Source: CAD feature listing. Evaluate the final solid. Frame: model axes, mm. Give positions to 0.01 mm unless a question says otherwise; leave off trailing zeros. Write each loop counter-clockwise with the first axis right and the second up, starting at its lowest first coordinate (ties: lowest second). Pieces come first, ordered by that corner, then holes. Notation, with made-up numbers: (-2, 9.25) - (4, 9.25) arc R9 ccw to (4, 17.25) - close; hole circle Ø10 at (-1, -20). An arc over 180 degrees is marked (long way). One line per question, with ' | ' between items. Start each with the question number.
(1) Ray query, line 1 (Z direction, x = 254.5, y = 0.7); line 2 (Z direction, x = 114, y = 0.5); line 3 (Z direction, x = 36, y = 0.6). Return the intervals inside material, ascending. Write a range as [from, to].
(2) Section A-A, the plane x = 193. Return loops of the section in (y, z).
(3) Section B-B, the plane y = 1.6. State how many separate pieces and enclosed holes the cut face has, plus the area to 3 significant figures.
```python
from build123d import *

# Parameters (mm, degrees)
SKETCH_1_R      = 1.5
SKETCH_1_W      = 18.5
SKETCH_1_H      = 18.5
SKETCH_1_W_2    = 17
SKETCH_1_H_2    = 17
EXTRUDE_1_DEPTH = 2


with BuildPart() as part:
    # 草图1 → 凸台-拉伸1 (new body)
    with BuildSketch(Plane(origin=(0, 0, 0), x_dir=(1, 0, 0), z_dir=(0, 1, 0))):
        with BuildLine():
            Line((10, 0), (136.884360712, 0))
            ThreePointArc((136.884360712, 0), (137.900113715, -0.277140216), (138.634360712, -1.031754163))
            Line((138.634360712, -1.031754163), (139.429147615, -2.468245837))
            ThreePointArc((139.429147615, -2.468245837), (140.163394612, -3.222859784), (141.179147615, -3.5))
            Line((141.179147615, -3.5), (143.5, -3.5))
            Line((143.5, -3.5), (166.5, -3.5))
            Line((166.5, -3.5), (168.820852385, -3.5))
            ThreePointArc((168.820852385, -3.5), (169.836605388, -3.222859784), (170.570852385, -2.468245837))
            Line((170.570852385, -2.468245837), (171.365639288, -1.031754163))
            ThreePointArc((171.365639288, -1.031754163), (172.099886285, -0.277140216), (173.115639288, 0))
            Line((173.115639288, 0), (300, 0))
            ThreePointArc((300, 0), (307.071067812, -2.928932188), (310, -10))
            Line((310, -10), (310, -210))
            ThreePointArc((310, -210), (307.071067812, -217.071067812), (300, -220))
            Line((300, -220), (10, -220))
            ThreePointArc((10, -220), (2.928932188, -217.071067812), (0, -210))
            Line((0, -210), (0, -10))
            ThreePointArc((0, -10), (2.928932188, -2.928932188), (10, 0))
        make_face()
        with Locations(Location((14, -14, 0), (0, 0, 270))):
            Circle(SKETCH_1_R, mode=Mode.SUBTRACT)
        with Locations(Location((14, -206, 0), (0, 0, 270))):
            Circle(SKETCH_1_R, mode=Mode.SUBTRACT)
        with Locations(Location((296, -206, 0), (0, 0, 270))):
            Circle(SKETCH_1_R, mode=Mode.SUBTRACT)
        with Locations(Location((296, -12.28568254, 0), (0, 0, 270))):
            Circle(SKETCH_1_R, mode=Mode.SUBTRACT)
        with Locations(Location((155, -206, 0), (0, 0, 270))):
            Circle(SKETCH_1_R, mode=Mode.SUBTRACT)
        with Locations(Location((175, -14, 0), (0, 0, 270))):
            Circle(SKETCH_1_R, mode=Mode.SUBTRACT)
        with Locations(Location((135, -14, 0), (0, 0, 270))):
            Circle(SKETCH_1_R, mode=Mode.SUBTRACT)
        with Locations(Location((296, -110, 0), (0, 0, 270))):
            Circle(SKETCH_1_R, mode=Mode.SUBTRACT)
        with Locations(Location((14, -110, 0), (0, 0, 270))):
            Circle(SKETCH_1_R, mode=Mode.SUBTRACT)
        with Locations(Location((155, -110, 0), (0, 0, 270))):
            Circle(SKETCH_1_R, mode=Mode.SUBTRACT)
        with Locations(Location((72, -110, 0), (0, 0, 270))):
            Circle(SKETCH_1_R, mode=Mode.SUBTRACT)
        with Locations(Location((72, -168.903225806, 0), (0, 0, 270))):
            Circle(SKETCH_1_R, mode=Mode.SUBTRACT)
        with Locations(Location((72, -51.096774194, 0), (0, 0, 270))):
            Circle(SKETCH_1_R, mode=Mode.SUBTRACT)
        with Locations(Location((42, -168.903225806, 0), (0, 0, 270))):
            Circle(SKETCH_1_R, mode=Mode.SUBTRACT)
        with Locations(Location((102, -168.903225806, 0), (0, 0, 270))):
            Circle(SKETCH_1_R, mode=Mode.SUBTRACT)
        with Locations(Location((238, -110, 0), (0, 0, 270))):
            Circle(SKETCH_1_R, mode=Mode.SUBTRACT)
        with Locations(Location((238, -168.903225806, 0), (0, 0, 270))):
            Circle(SKETCH_1_R, mode=Mode.SUBTRACT)
        with Locations(Location((268, -168.903225806, 0), (0, 0, 270))):
            Circle(SKETCH_1_R, mode=Mode.SUBTRACT)
        with Locations(Location((208, -168.903225806, 0), (0, 0, 270))):
            Circle(SKETCH_1_R, mode=Mode.SUBTRACT)
        with Locations(Location((246, -39, 0), (0, 0, 270))):
            Circle(SKETCH_1_R, mode=Mode.SUBTRACT)
        with Locations(Location((198, -39, 0), (0, 0, 270))):
            Circle(SKETCH_1_R, mode=Mode.SUBTRACT)
        with Locations(Location((110, -70, 0), (0, 0, 270))):
            Circle(SKETCH_1_R, mode=Mode.SUBTRACT)
        with Locations(Location((38, -51.096774194, 0), (0, 0, 270))):
            Circle(SKETCH_1_R, mode=Mode.SUBTRACT)
        with Locations(Location((198, -110, 0), (0, 0, 270))):
            Circle(SKETCH_1_R, mode=Mode.SUBTRACT)
        with Locations(Location((143.5, -90, 0), (0, 0, 270))):
            Circle(SKETCH_1_R, mode=Mode.SUBTRACT)
        with Locations((38, -24)):
            Rectangle(SKETCH_1_W, SKETCH_1_H, mode=Mode.SUBTRACT)
        with Locations((62, -24)):
            Rectangle(SKETCH_1_W, SKETCH_1_H, mode=Mode.SUBTRACT)
        with Locations((86, -24)):
            Rectangle(SKETCH_1_W, SKETCH_1_H, mode=Mode.SUBTRACT)
        with Locations((110, -24)):
            Rectangle(SKETCH_1_W, SKETCH_1_H, mode=Mode.SUBTRACT)
        with Locations((198, -24)):
            Rectangle(SKETCH_1_W, SKETCH_1_H, mode=Mode.SUBTRACT)
        with Locations((222, -24)):
            Rectangle(SKETCH_1_W, SKETCH_1_H, mode=Mode.SUBTRACT)
        with Locations((246, -24)):
            Rectangle(SKETCH_1_W, SKETCH_1_H, mode=Mode.SUBTRACT)
        with Locations((270, -24)):
            Rectangle(SKETCH_1_W, SKETCH_1_H, mode=Mode.SUBTRACT)
        with Locations((89, -53)):
            Rectangle(SKETCH_1_W_2, SKETCH_1_H_2, mode=Mode.SUBTRACT)
        with Locations((84, -77)):
            Rectangle(SKETCH_1_W_2, SKETCH_1_H_2, mode=Mode.SUBTRACT)
        with Locations((106, -90)):
            Rectangle(SKETCH_1_W_2, SKETCH_1_H_2, mode=Mode.SUBTRACT)
        with Locations((58, -80)):
            Rectangle(SKETCH_1_W_2, SKETCH_1_H_2, mode=Mode.SUBTRACT)
        with Locations((36, -97)):
            Rectangle(SKETCH_1_W_2, SKETCH_1_H_2, mode=Mode.SUBTRACT)
        with Locations((114, -130)):
            Rectangle(SKETCH_1_W_2, SKETCH_1_H_2, mode=Mode.SUBTRACT)
        with Locations((145, -138)):
            Rectangle(SKETCH_1_W_2, SKETCH_1_H_2, mode=Mode.SUBTRACT)
        with Locations((190, -130)):
            Rectangle(SKETCH_1_W_2, SKETCH_1_H_2, mode=Mode.SUBTRACT)
        with Locations((173, -85)):
            Rectangle(SKETCH_1_W_2, SKETCH_1_H_2, mode=Mode.SUBTRACT)
        with Locations((190, -66)):
            Rectangle(SKETCH_1_W_2, SKETCH_1_H_2, mode=Mode.SUBTRACT)
        with Locations((198, -90)):
            Rectangle(SKETCH_1_W_2, SKETCH_1_H_2, mode=Mode.SUBTRACT)
        with Locations((215, -58)):
            Rectangle(SKETCH_1_W_2, SKETCH_1_H_2, mode=Mode.SUBTRACT)
        with Locations((222, -84)):
            Rectangle(SKETCH_1_W_2, SKETCH_1_H_2, mode=Mode.SUBTRACT)
        with Locations((241, -58)):
            Rectangle(SKETCH_1_W_2, SKETCH_1_H_2, mode=Mode.SUBTRACT)
        with Locations((247, -84)):
            Rectangle(SKETCH_1_W_2, SKETCH_1_H_2, mode=Mode.SUBTRACT)
        with Locations((266, -66)):
            Rectangle(SKETCH_1_W_2, SKETCH_1_H_2, mode=Mode.SUBTRACT)
    extrude(amount=EXTRUDE_1_DEPTH)


solid = part.part
```
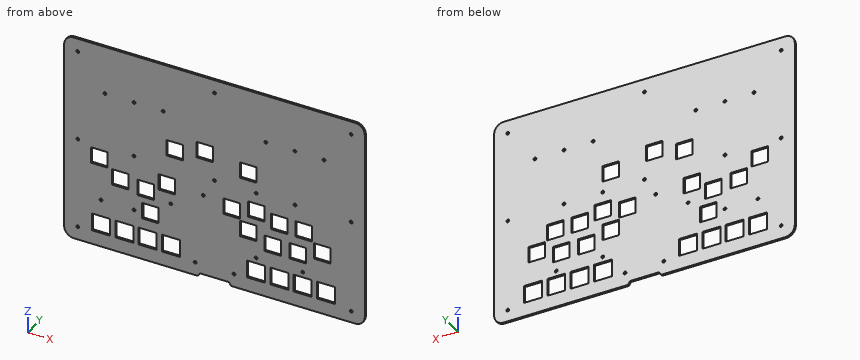
Check sheet entries:
1) line 1: [0, 14.75], [33.25, 75.5], [92.5, 220] | line 2: [0, 14.75], [33.25, 81.5], [98.5, 121.5], [138.5, 220] | line 3: [0, 14.75], [33.25, 88.5], [105.5, 220]
2) outline: (0, 0) - (2, 0) - (2, 14.75) - (0, 14.75) - close; (0, 33.25) - (2, 33.25) - (2, 57.5) - (0, 57.5) - close; (0, 74.5) - (2, 74.5) - (2, 81.5) - (0, 81.5) - close; (0, 98.5) - (2, 98.5) - (2, 121.5) - (0, 121.5) - close; (0, 138.5) - (2, 138.5) - (2, 220) - (0, 220) - close
3) separate pieces: 1 | enclosed holes: 49 | area: 60,500 mm²
